```python
from build123d import *

# Parameters (mm, degrees)
SKETCH1_R           = 4.5
SKETCH1_R_2         = 2.5
BOSS_EXTRUDE1_DEPTH = 19
SKETCH1_3_R         = 4.5
SKETCH1_3_R_2       = 2.5
SKETCH1_3_R_3       = 2.1
BOSS_EXTRUDE2_DEPTH = 1.6
SKETCH1_4_R         = 2.1
BOSS_EXTRUDE3_DEPTH = 0.8
SKETCH1_5_R         = 2.5
BOSS_EXTRUDE4_DEPTH = 4
BOSS_EXTRUDE5_DEPTH = 6
FILLET1_R           = 1
FILLET2_R           = 1


with BuildPart() as part:
    # Sketch1 → Boss-Extrude1 (new body)
    # profile 1 of 3: a face of its own
    with BuildSketch(Plane(origin=(0, 0, 0), x_dir=(1, 0, 0), z_dir=(0, 1, 0))):
        with BuildLine():
            ThreePointArc((10.911671632, 8.771283954), (-13.999968399, 0.029746015), (10.874300232, -8.817573048))
            Line((10.874300232, -8.817573048), (13.700622891, -8.817573048))
            Line((13.700622891, -8.817573048), (14.645115165, -7.3))
            Line((14.645115165, -7.3), (17.1, -7.3))
            Line((17.1, -7.3), (17.1, 7.3))
            Line((17.1, 7.3), (15.341903899, 7.3))
            Line((15.341903899, 7.3), (14.326809253, 8.771283954))
            Line((14.326809253, 8.771283954), (10.911671632, 8.771283954))
        make_face()
        with Locations((-8, 0)):
            Circle(SKETCH1_R, mode=Mode.SUBTRACT)
    # profile 2 of 3: a face of its own
    with BuildSketch(Plane(origin=(0, 0, 0), x_dir=(1, 0, 0), z_dir=(0, 1, 0))):
        with Locations((-8, 0)):
            Circle(SKETCH1_R)
        with Locations((-8, 0)):
            Circle(SKETCH1_R_2, mode=Mode.SUBTRACT)
    # profile 3 of 3: a face of its own
    with BuildSketch(Plane(origin=(0, 0, 0), x_dir=(1, 0, 0), z_dir=(0, 1, 0))):
        with Locations((-8, 0)):
            Circle(SKETCH1_R_2)
    extrude(amount=BOSS_EXTRUDE1_DEPTH)

    # Sketch1<3> → Boss-Extrude2 (add)
    # profile 1 of 2: a face of its own
    with BuildSketch(Plane(origin=(0, 0, 0), x_dir=(1, 0, 0), z_dir=(0, 1, 0))):
        with Locations(Location((-8, 0, 0), (0, 0, 270))):
            Circle(SKETCH1_3_R)
        with Locations(Location((-8, 0, 0), (0, 0, 270))):
            Circle(SKETCH1_3_R_2, mode=Mode.SUBTRACT)
    # profile 2 of 2: a face of its own
    with BuildSketch(Plane(origin=(0, 0, 0), x_dir=(1, 0, 0), z_dir=(0, 1, 0))):
        with Locations((0, 17.5)):
            Circle(SKETCH1_3_R_3)
    extrude(amount=-BOSS_EXTRUDE2_DEPTH)


with BuildPart() as boss_extrude2_kept_piece:
    # of the separate pieces the step leaves, the one the design keeps (boss_extrude2_pieces_kept)
    add(part.part.solids().sort_by_distance((10.911671632, 0, -8.771283954))[0])

    # Sketch1<4> → Boss-Extrude3 (add)
    # profile 1 of 2: a face of its own
    with BuildSketch(Plane(origin=(0, 0, 0), x_dir=(1, 0, 0), z_dir=(0, 1, 0))):
        with BuildLine():
            ThreePointArc((-3.5, 13.555441712), (0, 14), (3.5, 13.555441712))
            Line((3.5, 13.555441712), (3.5, 17.5))
            ThreePointArc((3.5, 17.5), (0, 21), (-3.5, 17.5))
            Line((-3.5, 17.5), (-3.5, 13.555441712))
        make_face()
        with Locations(Location((0, 17.5, 0), (0, 0, 270))):
            Circle(SKETCH1_4_R, mode=Mode.SUBTRACT)
    # profile 2 of 2: a face of its own
    with BuildSketch(Plane(origin=(0, 0, 0), x_dir=(1, 0, 0), z_dir=(0, 1, 0))):
        with BuildLine():
            ThreePointArc((3.5, -13.555441712), (0, -14), (-3.5, -13.555441712))
            Line((-3.5, -13.555441712), (-3.5, -17.5))
            ThreePointArc((-3.5, -17.5), (0, -21), (3.5, -17.5))
            Line((3.5, -17.5), (3.5, -13.555441712))
        make_face()
        with Locations(Location((0, -17.5, 0), (0, 0, 270))):
            Circle(SKETCH1_4_R, mode=Mode.SUBTRACT)
    extrude(amount=BOSS_EXTRUDE3_DEPTH)

    # Sketch1<5> → Boss-Extrude4 (add)
    with BuildSketch(Plane(origin=(0, 0, 0), x_dir=(1, 0, 0), z_dir=(0, 1, 0))):
        with Locations(Location((-8, 0, 0), (0, 0, 270))):
            Circle(SKETCH1_5_R)
    extrude(amount=-BOSS_EXTRUDE4_DEPTH)

    # Sketch5 → Boss-Extrude5 (add)
    with BuildSketch(Plane.XZ.offset(4)):
        with BuildLine():
            Line((-9.968251002, 1.283884289), (-10.145143616, 1.283884289))
            ThreePointArc((-10.145143616, 1.283884289), (-10.5, 0), (-10.145143616, -1.283884289))
            Line((-10.145143616, -1.283884289), (-9.968251002, -1.283884289))
            Line((-9.968251002, -1.283884289), (-9.968251002, 1.283884289))
        make_face()
        with BuildLine():
            Line((-5.854856384, 1.283884289), (-9.968251002, 1.283884289))
            Line((-9.968251002, 1.283884289), (-9.968251002, -1.283884289))
            Line((-9.968251002, -1.283884289), (-5.854856384, -1.283884289))
            ThreePointArc((-5.854856384, -1.283884289), (-5.590346598, -0.666010871), (-5.5, 0))
            ThreePointArc((-5.5, 0), (-5.590346598, 0.666010871), (-5.854856384, 1.283884289))
        make_face()
    extrude(amount=BOSS_EXTRUDE5_DEPTH)

    # Fillet1
    # the kernel refuses this fillet: 1 mm, written as the material it adds along each edge
    with BuildSketch(Plane(origin=(-12.645143616, -4, 1.283884289), x_dir=(0, 0, 1), z_dir=(1, 0, 0))) as fillet1_piece_1_section:
        with BuildLine():
            CenterArc((FILLET1_R, FILLET1_R), FILLET1_R, 180, 90)
            Line((0, FILLET1_R), (0, 0))
            Line((0, 0), (FILLET1_R, 0))
        make_face()
    fillet1_piece_1 = extrude(amount=9.290287231, mode=Mode.PRIVATE)
    fillet1_piece_1 = fillet1_piece_1 & Plane(origin=(-8, -4.238121926, 0), x_dir=(0, 0, 1), z_dir=(0, 1, 0)) * Cylinder(2.5, 23, mode=Mode.PRIVATE)
    add(fillet1_piece_1)

    # Fillet2
    # the kernel refuses this fillet: 1 mm, written as the material it adds along each edge
    with BuildSketch(Plane(origin=(-12.645143616, -4, -1.283884289), x_dir=(0, -1, 0), z_dir=(1, 0, 0))) as fillet2_piece_1_section:
        with BuildLine():
            CenterArc((FILLET2_R, FILLET2_R), FILLET2_R, 180, 90)
            Line((0, FILLET2_R), (0, 0))
            Line((0, 0), (FILLET2_R, 0))
        make_face()
    fillet2_piece_1 = extrude(amount=9.290287231, mode=Mode.PRIVATE)
    fillet2_piece_1 = fillet2_piece_1 & Plane(origin=(-8, -4.238121979, 0), x_dir=(-0.8580574462690832, 0, 0.5135537156930905), z_dir=(0, 1, 0)) * Cylinder(2.5, 23, mode=Mode.PRIVATE)
    add(fillet2_piece_1)


solid = boss_extrude2_kept_piece.part
```
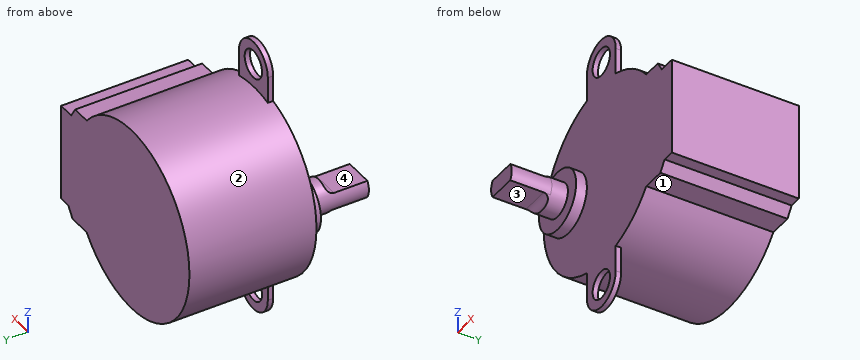
For this review, take the finished solid that the model builds, in its own axes (mm). Face numbers are marked on the shaded views. A direction names the side the tool comes from. Round coordinates to 2 decimals unless told otherwise and drop trailing zeros. Write each loop counter-clockwise with the first axis right and the second up, starting at its lowest first coordinate (ties: lowest second). Pieces come first, ordered by that corner, then holes. Notation, with made-up numbers: (-36.5, -37.5) -> (11.5, -37.5) arc R13 cw to (11.5, -24.5) -> close; hole circle Ø10 at (88.25, 70.25). An arc over 180 degrees is marked (long way). Use one line per item in the form item = value.
1) Take a section at B-B, the plane z = 0. Write out the cut boundary in (x, y), and give its area (3 significant figures).
Found:
outline = (-14, 0) -> (-12.5, 0) -> (-12.5, -1.6) -> (-10.5, -1.6) -> (-10.5, -10) -> (-5.5, -10) -> (-5.5, -1.6) -> (-3.5, -1.6) -> (-3.5, 0) -> (17.1, 0) -> (17.1, 19) -> (-14, 19) -> close
area = 647 mm2
2) Clearance check with flat-ended pins moving along their axes: pin 1 (8 mm diameter, centred on y = 9.5, z = -16.5, fed in from +X); pin 2 (0.9 mm diameter, centred on y = 0.5, z = -15, fed in from -X); pin 3 (2 mm diameter, centred on x = -8, y = -7, fed in from +Z); pin 4 (4 mm diameter, centred on x = 0, z = 17.5, fed in from -Y). State where each tip first meets the part, or that it passes through.
Found:
pin_1 = 6.3
pin_2 = -3.5
pin_3 = 1.28
pin_4 = through
3) Tool access review of the marked faces 1, 2, 3 and 4: name each direction out of +Z, -Z, +X, -X, +Y, -Y from which nothing blocks a thin tool from reaching the whole face with its end or side.
Found:
face_1 = -Z, +X, +Y, -Y
face_2 = +Y
face_3 = -Z, +X, -X, -Y
face_4 = +Z, +X, -X, -Y
4) Take a section at A-A, the plane x = 0. Write out the cut boundary in (y, z), and give its area (3 significant figures).
Found:
outline = (0, -21) -> (0.8, -21) -> (0.8, -19.6) -> (0, -19.6) -> close; (0, -15.4) -> (0.8, -15.4) -> (0.8, -14) -> (19, -14) -> (19, 14) -> (0.8, 14) -> (0.8, 15.4) -> (0, 15.4) -> close; (0, 19.6) -> (0.8, 19.6) -> (0.8, 21) -> (0, 21) -> close
area = 536 mm2
5) To check wall thickness, follow L1, parallel to X at y = 0.2, z = 17.5; L2, parallel to Y at x = 15, z = -3; L3, parallel to Z at x = 3.5, y = 5.75. State the ranges of each line that lie inside material, in increasing order. Write a range as from..to.
Found:
L1 = -3.5..-2.1, 2.1..3.5
L2 = 0..19
L3 = -13.56..13.56
6) Take a section at C-C, the plane y = 6. Write out the cut boundary in (x, z), and give its area (3 significant figures).
Found:
outline = (10.87, 8.82) arc R14 ccw (long way) to (10.91, -8.77) -> (14.33, -8.77) -> (15.34, -7.3) -> (17.1, -7.3) -> (17.1, 7.3) -> (14.65, 7.3) -> (13.7, 8.82) -> close
area = 680 mm2
7) Take a section at D-D, the plane z = 16.5. Write out the cut boundary in (x, y), and give its area (3 significant figures).
Found:
outline = (-3.5, 0) -> (-1.85, 0) -> (-1.85, 0.8) -> (-3.5, 0.8) -> close; (1.85, 0) -> (3.5, 0) -> (3.5, 0.8) -> (1.85, 0.8) -> close
area = 2.65 mm2
